from build123d import *

# Parameters (mm, degrees)
BOSS_EXTRUDE1_DEPTH = 30
SKETCH2_R           = 8.5
CUT_EXTRUDE1_DEPTH  = 179
LPATTERN1_COUNT     = 2
LPATTERN1_PITCH     = 150
SKETCH3_R           = 2.5
CUT_EXTRUDE2_DEPTH  = 15
LPATTERN2_COUNT     = 2
LPATTERN2_PITCH     = 83
SKETCH4_R           = 6
CUT_EXTRUDE3_DEPTH  = 31
SKETCH5_R           = 8
CUT_EXTRUDE4_DEPTH  = 40


with BuildPart() as part:
    # Sketch1 → Boss-Extrude1 (new body)
    with BuildSketch(Plane.XY):
        with BuildLine():
            Line((0, 0), (0, 340))
            Line((0, 340), (178, 340))
            Line((178, 340), (178, 202.5))
            ThreePointArc((178, 202.5), (145.5, 170), (178, 137.5))
            Line((178, 137.5), (178, 30))
            Line((178, 30), (218, 30))
            Line((218, 30), (218, 0))
            Line((218, 0), (0, 0))
        make_face()
    extrude(amount=BOSS_EXTRUDE1_DEPTH)

    # Sketch2 → Cut-Extrude1 (cut, through all)
    with BuildSketch(Plane(origin=(178, 0, 0), x_dir=(0, 0, -1), z_dir=(1, 0, 0))):
        with Locations((-15, 95)):
            Circle(SKETCH2_R)
    cut_extrude1 = extrude(amount=-CUT_EXTRUDE1_DEPTH, mode=Mode.SUBTRACT)

    # LPattern1: Cut-Extrude1 ×2
    with Locations(*[(0, i * LPATTERN1_PITCH, 0) for i in range(1, LPATTERN1_COUNT)]):
        add(cut_extrude1, mode=Mode.SUBTRACT)

    # Sketch3 → Cut-Extrude2 (cut)
    with BuildSketch(Plane(origin=(178, 0, 0), x_dir=(0, 0, -1), z_dir=(1, 0, 0))):
        with Locations((-15, 128.5)):
            Circle(SKETCH3_R)
    cut_extrude2 = extrude(amount=-CUT_EXTRUDE2_DEPTH, mode=Mode.SUBTRACT)

    # LPattern2: Cut-Extrude2 ×2
    with Locations(*[(0, i * LPATTERN2_PITCH, 0) for i in range(1, LPATTERN2_COUNT)]):
        add(cut_extrude2, mode=Mode.SUBTRACT)

    # Sketch4 → Cut-Extrude3 (cut, through all)
    with BuildSketch(Plane(origin=(0, 30, 0), x_dir=(1, 0, 0), z_dir=(0, 1, 0))):
        with Locations((198, -15)):
            Circle(SKETCH4_R)
    extrude(amount=-CUT_EXTRUDE3_DEPTH, mode=Mode.SUBTRACT)

    # Sketch5 → Cut-Extrude4 (cut)
    with BuildSketch(Plane(origin=(0, 340, 0), x_dir=(1, 0, 0), z_dir=(0, 1, 0))):
        with Locations((20, -15)):
            Circle(SKETCH5_R)
        with Locations((143, -15)):
            Circle(SKETCH5_R)
    extrude(amount=-CUT_EXTRUDE4_DEPTH, mode=Mode.SUBTRACT)


solid = part.part
Input: part model. Units: mm. Frame: model coordinates. A direction names the side the tool comes from. Give positions to 0.01 mm unless a question says otherwise; leave off trailing zeros. Order: outer loops, then holes, each group sorted by start corner. A loop starts at its lowest first (then second) coordinate and runs counter-clockwise, first axis right, second up. Notation, with made-up numbers: M 10.25,18.25 L 66.25,18.25 A22 ccw 66.25,33.25 Z; hole C -23,60 d9. An arc over 180 degrees is marked long. Answer as a JSON object with one key per item and string values.
1. Pull-direction query (Z, two-part tool) for faces 1 (the flat face through (178, 85, 15)), 2 (the flat face through (86, 172, 0)), 3 (the flat face through (20, 300, 15)); classes: +Z half, -Z half, draft (parallel to the pull), parting line (faces both ways), or undercut.
Result sheet:
{"face 1": "draft", "face 2": "-Z half", "face 3": "undercut"}
2. Cut plane A-A, the plane y = 95. Output: boundary loops of the cut face in (x, z).
Result sheet:
{"outline": "M 0,0 L 178,0 L 178,6.5 L 0,6.5 Z; M 0,23.5 L 178,23.5 L 178,30 L 0,30 Z"}
3. Reachability of faces 4 (the cylindrical face through (12, 320, 15)), 5 (the flat face through (0, 168, 15)), 6 (the flat face through (198, 30, 8)) from +Z, -Z, +X, -X, +Y, -Y: full face, straight path, thin tool, end or side. Return the list, or none.
Result sheet:
{"face 4": "+Y", "face 5": "+Z, -Z, -X, +Y, -Y", "face 6": "+Z, -Z, +X, +Y"}
4. Ray query, line 1 (Y direction, x = 21, z = 16); line 2 (Y direction, x = 123, z = 15); line 3 (X direction, y = 324.5, z = 15). Return the intervals inside material, ascending. Write a range as [from, to].
Result sheet:
{"line 1": "[0, 86.56], [103.44, 236.56], [253.44, 300]", "line 2": "[0, 86.5], [103.5, 236.5], [253.5, 340]", "line 3": "[0, 12], [28, 135], [151, 178]"}
5. Cut plane B-B, the plane x = 31.5. Output: boundary loops of the cut face in (y, z), and give its area (3 significant figures).
Result sheet:
{"outline": "M 0,0 L 340,0 L 340,30 L 0,30 Z; hole C 95,15 d17; hole C 245,15 d17", "area": "9,750 mm²"}
6. First-contact query: P1, Ø5, axis at x = 140, z = 13, coming from the +Y side; P2, Ø15, axis at y = 57.5, z = 16, coming from the +X side; P3, Ø15, axis at x = 193.5, z = 19.5, coming from the +Y side. Flat tips, straight axial feed; report the tip coordinate or a pass-through.
Result sheet:
{"P1": "y = 300", "P2": "x = 178", "P3": "y = 30"}
